```python
from build123d import *

# Parameters (mm, degrees)
F1_DEPTH = 6.35
F2_W     = 31.75
F2_H     = 63.1597361455
F2_W_2   = 80.4999943972
F2_H_2   = 31.75
F2_W_3   = 22.4999943972
F3_DEPTH = 6.35
F4_W     = 19.05
F4_H     = 89.0185771326
F4_W_2   = 92.1357582898
F4_H_2   = 19.05
F5_DEPTH = 6.35
F6_R     = 25.4
F7_R     = 6.35


with BuildPart() as f1:
    # F0 (on Top) → F1 (new body)
    with BuildSketch(Plane.XY):
        with BuildLine():
            Line((-45, 95), (-189, 95))
            Line((-189, 95), (-189, -170))
            Line((-189, -170), (131, -170))
            Line((131, -170), (131, 95))
            Line((131, 95), (45, 95))
            Line((45, 95), (45, 0))
            ThreePointArc((45, 0), (0, -45), (-45, 0))
            Line((-45, 0), (-45, 95))
        make_face()
        with BuildLine():
            Line((-76.7500028014, 63.2499971986), (-76.7500028014, 0))
            ThreePointArc((-76.7500028014, 0), (0, -76.7500028014), (76.7500028014, 0))
            Line((76.7500028014, 0), (76.7500028014, 63.2499971986))
            Line((76.7500028014, 63.2499971986), (99.2499971986, 63.2499971986))
            Line((99.2499971986, 63.2499971986), (99.2499971986, -138.2499971986))
            Line((99.2499971986, -138.2499971986), (-157.2499971986, -138.2499971986))
            Line((-157.2499971986, -138.2499971986), (-157.2499971986, 63.2499971986))
            Line((-157.2499971986, 63.2499971986), (-76.7500028014, 63.2499971986))
        make_face(mode=Mode.SUBTRACT)
    extrude(amount=-F1_DEPTH)

    # F2 (on face) → F3 (join)
    with BuildSketch(Plane.XY):
        with Locations((0, -106.6701291258)):
            Rectangle(F2_W, F2_H)
        with Locations((-117, 15.875)):
            Rectangle(F2_W_2, F2_H_2)
        with Locations((88, 15.875)):
            Rectangle(F2_W_3, F2_H_2)
        Polygon((-46.2363796826, -61.2597757412), (-67.0740856459, -37.3045568904), (-157.2499971986, -115.7450479419), (-157.2499971986, -138.2499971986), (-134.7450479419, -138.2499971986), align=None)
        Polygon((55.8022859826, -52.6940965302), (29.7003793774, -70.7704062081), (76.4319075424, -138.2499971986), (99.2499971986, -138.2499971986), (99.2499971986, -115.4319075424), align=None)
    extrude(amount=-F3_DEPTH)

    # F4 (on face) → F5 (join)
    with BuildSketch(Plane.XY):
        with Locations((-117, -44.5092885663)):
            Rectangle(F4_W, F4_H)
        with Locations((-61.9428791449, -105.4698864699)):
            Rectangle(F4_W_2, F4_H_2)
    extrude(amount=-F5_DEPTH)

    # F6
    f6_edges = [f1.edges().sort_by_distance(p)[0] for p in [
        (-189, 95, -3.175),
        (-189, -170, -3.175),
        (131, -170, -3.175),
        (131, 95, -3.175),
        (45, 95, -3.175),
        (-45, 95, -3.175),
    ]]
    fillet(f6_edges, radius=F6_R)

    # F7
    f7_edges = [f1.edges().sort_by_distance(p)[0] for p in [
        (76.750003, 63.249997, -3.175),
        (99.249997, 63.249997, -3.175),
        (76.750003, 31.75, -3.175),
        (99.249997, 31.75, -3.175),
        (55.802286, -52.694097, -3.175),
        (-157.249997, 31.75, -3.175),
        (-134.745048, -138.249997, -3.175),
        (-86.110703, -95.944886, -3.175),
        (15.875, -138.249997, -3.175),
        (-157.249997, 0, -3.175),
        (-157.249997, 63.249997, -3.175),
        (-107.475, 0, -3.175),
        (-46.23638, -61.259776, -3.175),
        (-108.010758, -114.994886, -3.175),
        (15.875, -75.090261, -3.175),
        (76.750003, 0, -3.175),
        (-76.750003, 31.75, -3.175),
        (-67.074086, -37.304557, -3.175),
        (-15.875, -95.944886, -3.175),
        (76.431908, -138.249997, -3.175),
        (-15.875, -138.249997, -3.175),
        (-126.525, -89.018577, -3.175),
        (-107.475, -72.447729, -3.175),
        (-157.249997, -115.745048, -3.175),
        (99.249997, 0, -3.175),
        (-15.875, -75.090261, -3.175),
        (-15.875, -114.994886, -3.175),
        (-76.750003, 0, -3.175),
        (-76.750003, 63.249997, -3.175),
        (29.700379, -70.770406, -3.175),
        (-126.525, 0, -3.175),
        (99.249997, -115.431908, -3.175),
    ]]
    fillet(f7_edges, radius=F7_R)


solid = f1.part
```
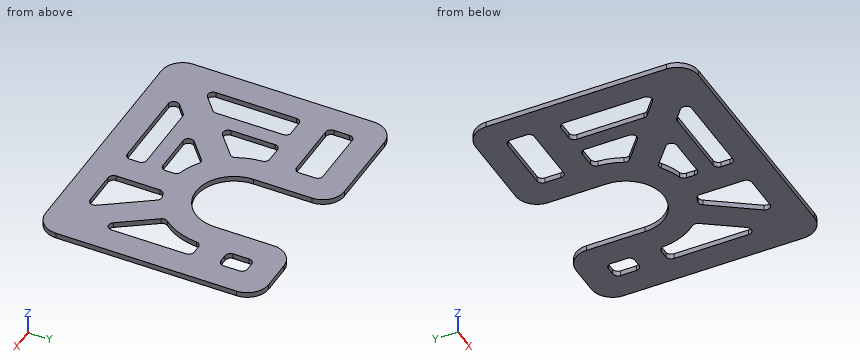
The model under review builds one solid part; all positions refer to its coordinate system, in mm. Round coordinates to 2 decimals unless told otherwise and drop trailing zeros. Write each loop counter-clockwise with the first axis right and the second up, starting at its lowest first coordinate (ties: lowest second). Pieces come first, ordered by that corner, then holes. Notation, with made-up numbers: (32.25, 7) - (51.25, 7) arc R18 cw to (51.25, 25) - close; hole circle Ø3 at (-25.5, -29). An arc over 180 degrees is marked (long way). One line per question, with ' | ' between items.
Item 1: Add section B-B, the plane z = -3. State how many separate pieces and enclosed holes the cut face has, then the cut area to 3 significant figures.
Resolved:
separate pieces: 1 | enclosed holes: 8 | area: 55,100 mm2
Item 2: Add section C-C, the plane x = 0. Give the boundary of the cut face in (y, z).
Resolved:
outline: (-170, -6.35) - (-45, -6.35) - (-45, 0) - (-170, 0) - close
Item 3: To check wall thickness, follow probe 1 along Y at (x, z) = (-116, -1); probe 2 along Y at (x, z) = (-150, -1.75); probe 3 along X at (y, z) = (38, -1). State the ranges of each line that lie inside material, in increasing order.
Resolved:
probe 1: y = -170 to -138.25, -121.94 to 31.75, 63.25 to 95 | probe 2: y = -170 to -108.09, 0 to 31.75, 63.25 to 95 | probe 3: x = -189 to -157.25, -76.75 to -45, 45 to 76.75, 99.25 to 131
Item 4: Add section A-A, the plane y = 17. Give the boundary of the cut face in (x, z).
Resolved:
outline: (-189, -6.35) - (-45, -6.35) - (-45, 0) - (-189, 0) - close; (45, -6.35) - (131, -6.35) - (131, 0) - (45, 0) - close
